Source: CAD feature listing. Evaluate the final solid. Frame: model axes, mm. A direction names the side the tool comes from. Round coordinates to 2 decimals unless told otherwise and drop trailing zeros. Order: outer loops, then holes, each group sorted by start corner. A loop starts at its lowest first (then second) coordinate and runs counter-clockwise, first axis right, second up. Notation, with made-up numbers: M 61,31.5 L 77,31.5 A33 ccw 77,68.5 Z; hole C -31,-4 d8. An arc over 180 degrees is marked long. Use one line per item in the form item = value. Start each with the question number.
Q1. Section B-B (x = 0). Return the cut outline in (y, z).
Q2. Section C-C (y = -10.75). Return the cut outline in (x, z).
Q3. Contact query for flat-ended pins moving along their axis: pin 1 (14.5 mm diameter, centred on x = 1.5, z = 9.5, fed in from -Y); pin 2 (5 mm diameter, centred on x = -1, y = -2, fed in from -Z); pin 3 (3 mm diameter, centred on y = -6, z = 18.5, fed in from -X). Output: stop coordinate, or through.
Q4. Pull-direction query (X, two-part tool) for faces 1 (the cylindrical face through (0.867, -1.055, -3.905)), 2 (the cylindrical face through (29.97, -9.72, -1.32)), 3 (the flat face through (-9, -14.3, 27)); classes: pulls with the +X half, pulls with the -X half, needs draft (parallel to the pull), parting line crosses it, or undercut.
Q5. Material intervals for probe 1 along X at (y, z) = (-9, 0); probe 2 along Y at (x, z) = (2.5, -7.5), sorted ascending.
Q6. Reachability of faces 4 (the flat face through (0, 0, 5)), 5 (the cylindrical face through (22.11, -10.16, 16.95)) from +Z, -Z, +X, -X, +Y, -Y: full face, straight path, thin tool, end or side. Return the list, or none.
Q7. Section A-A (z = 0). Return the cut outline in (x, y), plus the area to 3 significant figures.
from build123d import *

# Parameters (mm, degrees)
ENL_V_MAT_EXTRU_1_REACH = 46.772
ESQUISSE3_R             = 4


with BuildPart() as part:
    # Esquisse2 → Révolution1 (revolve)
    with BuildSketch(Plane.XY):
        with BuildLine():
            Line((0, 0), (-25, 0))
            ThreePointArc((-25, 0), (-28.535533906, -1.464466094), (-30, -5))
            Line((-30, -5), (-30, -14.3))
            Line((-30, -14.3), (-27.86, -14.3))
            Line((-27.86, -14.3), (-27.86, -6.14))
            ThreePointArc((-27.86, -6.14), (-26.688427125, -3.311572875), (-23.86, -2.14))
            Line((-23.86, -2.14), (0, -2.14))
            Line((0, -2.14), (0, 0))
        make_face()
    revolve(axis=Axis((0, 0, 0), (0, -1, 0)))

    # Esquisse3 → Enlèv. mat.-Extru.1 (cut, up to next)
    with BuildSketch(Plane(origin=(0, 0, 0), x_dir=(1, 0, 0), z_dir=(0, 1, 0)), mode=Mode.PRIVATE) as enl_v_mat_extru_1_sk1:
        with Locations(Location((0, 0, 0), (0, 0, 180))):
            Circle(ESQUISSE3_R)
    enl_v_mat_extru_1_tool1 = extrude(enl_v_mat_extru_1_sk1.sketch, amount=-ENL_V_MAT_EXTRU_1_REACH, mode=Mode.PRIVATE) & part.part
    add(enl_v_mat_extru_1_tool1.solids().sort_by_distance((0, 0, 0))[0], mode=Mode.SUBTRACT)


solid = part.part
Results list:
q1.outline = M -14.3,-30 L -5,-30 A5 ccw 0,-25 L 0,-4 L -2.14,-4 L -2.14,-23.86 A4 cw -6.14,-27.86 L -14.3,-27.86 Z; M -14.3,27.86 L -6.14,27.86 A4 cw -2.14,23.86 L -2.14,4 L 0,4 L 0,25 A5 ccw -5,30 L -14.3,30 Z
q2.outline = C 0,0 d60; hole C 0,0 d55.72
q3.pin_1 = -2.14
q3.pin_2 = -29.97
q3.pin_3 = -24.72
q4.face_1 = undercut
q4.face_2 = parting line crosses it
q4.face_3 = needs draft
q5.probe_1 = -30 to -27.86, 27.86 to 30
q5.probe_2 = -2.14 to 0
q6.face_4 = +Z, -Z, +X, -X, +Y
q6.face_5 = -Y
q7.outline = M -30,-14.3 L -27.86,-14.3 L -27.86,-6.14 A4 cw -23.86,-2.14 L -4,-2.14 L -4,0 L -25,0 A5 ccw -30,-5 Z; M 4,-2.14 L 23.86,-2.14 A4 cw 27.86,-6.14 L 27.86,-14.3 L 30,-14.3 L 30,-5 A5 ccw 25,0 L 4,0 Z
q7.area = 159 mm2
